Build history of the part. All positions in model axes, mm. Round coordinates to 2 decimals unless told otherwise and drop trailing zeros. Order: outer loops, then holes, each group sorted by start corner. A loop starts at its lowest first (then second) coordinate and runs counter-clockwise, first axis right, second up. Notation, with made-up numbers: (71, 6.25) -> (89, 6.25) arc R10 ccw to (89, 12.25) -> close; hole circle Ø4 at (80, 12). An arc over 180 degrees is marked (long way). Answer as CSV lines item,"result". Start each with the question number.
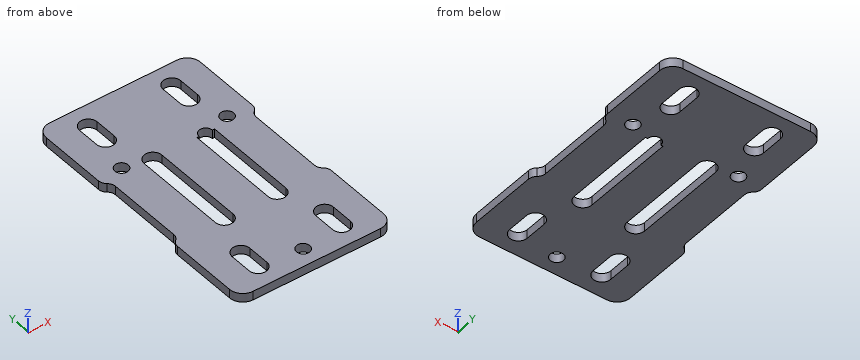
```python
from build123d import *

# Parameters (mm, degrees)
F0_R        = 1.5
F1_DEPTH    = 2
F2_R        = 3
F3_W        = 4
F3_H        = 5
F3_W_2      = 1.5
F3_H_2      = 21
F4_DEPTH    = 2.001
F5_R        = 2
F5_R_2      = 1.5
F6_DEPTH    = 2.001
F7_T1_DEPTH = 2
F8_R        = 2


# Not quite as in the source:
# - a fillet or chamfer that OpenCascade refuses, or shapes differently, is made with other operations: its cross-section is extruded or revolved along the edge and cut away or added


with BuildPart() as f1:
    # F0 (on Top) → F1 (new body)
    with BuildSketch(Plane.XY):
        Polygon((-17.5, 17.5), (-17.5, -17.5), (-17.5, -30), (17.5, -30), (17.5, -17.5), (17.5, 17.5), (17.5, 30), (-17.5, 30), align=None)
        with Locations((0, -26)):
            Circle(F0_R, mode=Mode.SUBTRACT)
        with Locations((-12, 12)):
            Circle(F0_R, mode=Mode.SUBTRACT)
        with Locations((12, 12)):
            Circle(F0_R, mode=Mode.SUBTRACT)
    extrude(amount=F1_DEPTH)

    # F2
    f2_edges = [f1.edges().sort_by_distance(p)[0] for p in [
        (-17.5, -30, 1),
        (17.5, -30, 1),
        (17.5, 30, 1),
        (-17.5, 30, 1),
    ]]
    fillet(f2_edges, radius=F2_R)

    # F3 (on face) → F4 (cut, through all)
    with BuildSketch(Plane.XY.offset(2)):
        with Locations((9.5, 22.5)):
            Rectangle(F3_W, F3_H)
        with Locations((9.5, -22.5)):
            Rectangle(F3_W, F3_H)
        with Locations((-9.5, -22.5)):
            Rectangle(F3_W, F3_H)
        with Locations((-9.5, 22.5)):
            Rectangle(F3_W, F3_H)
        with Locations((-16.75, 0)):
            Rectangle(F3_W_2, F3_H_2)
        with Locations((16.75, 0)):
            Rectangle(F3_W_2, F3_H_2)
        with Locations((-6, 0)):
            Rectangle(F3_W, F3_H_2)
        with Locations((6, 0)):
            Rectangle(F3_W, F3_H_2)
    extrude(amount=-F4_DEPTH, mode=Mode.SUBTRACT)

    # F5 (on face) → F6 (cut, through all)
    with BuildSketch(Plane.XY.offset(2)):
        with Locations((-9.5, 25)):
            Circle(F5_R)
        with Locations((9.5, 25)):
            Circle(F5_R)
        with Locations((9.5, -25)):
            Circle(F5_R)
        with Locations((-9.5, -25)):
            Circle(F5_R)
        with Locations((-9.5, -20)):
            Circle(F5_R)
        with Locations((9.5, -20)):
            Circle(F5_R)
        with Locations((6, -10.5)):
            Circle(F5_R)
        with Locations((-6, -10.5)):
            Circle(F5_R)
        with Locations((-6, 10.5)):
            Circle(F5_R)
        with Locations((6, 10.5)):
            Circle(F5_R_2)
        with Locations((9.5, 20)):
            Circle(F5_R)
        with Locations((-9.5, 20)):
            Circle(F5_R)
    extrude(amount=-F6_DEPTH, mode=Mode.SUBTRACT)

    # F7: fillet of radius 2 on 4 edges, made by hand

    # F7_s2 → F7_t1 (join)
    with BuildSketch(Plane.XY):
        with BuildLine():
            ThreePointArc((-17.5, -10.5), (-16.4188611699, -9.7882531983), (-16, -8.5635083269))
            Line((-16, -8.5635083269), (-16, -10.5))
            Line((-16, -10.5), (-17.5, -10.5))
        make_face()
        with BuildLine():
            ThreePointArc((-17.5, 10.5), (-16.4188611699, 9.7882531983), (-16, 8.5635083269))
            Line((-16, 8.5635083269), (-16, 10.5))
            Line((-16, 10.5), (-17.5, 10.5))
        make_face()
        with BuildLine():
            ThreePointArc((16, 8.5635083269), (16.4188611699, 9.7882531983), (17.5, 10.5))
            Line((17.5, 10.5), (16, 10.5))
            Line((16, 10.5), (16, 8.5635083269))
        make_face()
        with BuildLine():
            ThreePointArc((17.5, -10.5), (16.4188611699, -9.7882531983), (16, -8.5635083269))
            Line((16, -8.5635083269), (16, -10.5))
            Line((16, -10.5), (17.5, -10.5))
        make_face()
    extrude(amount=F7_T1_DEPTH)

    # F8
    f8_edges = [f1.edges().sort_by_distance(p)[0] for p in [
        (17.5, -10.5, 1),
        (17.5, 10.5, 1),
        (-17.5, -10.5, 1),
        (-17.5, 10.5, 1),
    ]]
    fillet(f8_edges, radius=F8_R)


solid = f1.part
```
Q1. Slice it at A-A, the plane x = -9.5. Write the cut outline in (y, z), plus the area to 3 significant figures.
Q2. Slice it at C-C, the plane y = 5. Write the cut outline in (x, z).
Q3. Slice it at B-B, the plane x = 0. Write the cut outline in (y, z), plus the area to 3 significant figures.
Q4. Slice it at D-D, the plane x = -6. Write the cut outline in (y, z), plus the area to 3 significant figures.
Q5. Flat gauge pin, fed straight in: pin 1 Ø12 at (x, y) = (8.5, 19.5) entering from -Z. Where does the tip first touch, or does it go through?
Q6. Probe L1, parallel to X at y = 2.5, z = 1.95; L2, parallel to Y at x = 9.5, z = 1.6; L3, parallel to X at y = 25, z = 1.4. List the from-to ranges inside material, lowest first.
Solutions:
1,outline,"(-30, 0) -> (-27, 0) -> (-27, 2) -> (-30, 2) -> close; (-18, 0) -> (18, 0) -> (18, 2) -> (-18, 2) -> close; (27, 0) -> (30, 0) -> (30, 2) -> (27, 2) -> close"
1,area,"84.0 mm2"
2,outline,"(-16, 0) -> (-8, 0) -> (-8, 2) -> (-16, 2) -> close; (-4, 0) -> (4, 0) -> (4, 2) -> (-4, 2) -> close; (8, 0) -> (16, 0) -> (16, 2) -> (8, 2) -> close"
3,outline,"(-30, 0) -> (-27.5, 0) -> (-27.5, 2) -> (-30, 2) -> close; (-24.5, 0) -> (30, 0) -> (30, 2) -> (-24.5, 2) -> close"
3,area,"114 mm2"
4,outline,"(-30, 0) -> (-12.5, 0) -> (-12.5, 2) -> (-30, 2) -> close; (12.5, 0) -> (30, 0) -> (30, 2) -> (12.5, 2) -> close"
4,area,"70.0 mm2"
5,pin 1,"stops at z = 0"
6,L1,"x = -16 to -8, -4 to 4, 8 to 16"
6,L2,"y = -30 to -27, -18 to 18, 27 to 30"
6,L3,"x = -17.5 to -11.5, -7.5 to 7.5, 11.5 to 17.5"
